The model under review builds one solid part; all positions refer to its coordinate system, in mm. A direction names the side the tool comes from. Round coordinates to 2 decimals unless told otherwise and drop trailing zeros. Order: outer loops, then holes, each group sorted by start corner. A loop starts at its lowest first (then second) coordinate and runs counter-clockwise, first axis right, second up. Notation, with made-up numbers: M -24,2.5 L 9,2.5 A23 cw 9,39.5 Z; hole C -8,76.5 d2. An arc over 180 degrees is marked long. Answer as a JSON object with one key per item and string values. Group by question number.
1. Add section A-A on z = 0.5. State the section outline as (x, y) points.
2. Clearance check with flat-ended pins moving along their axes: P1, Ø1.5, axis at x = 0, y = 12.73, coming from the +Z side; P2, Ø6.5, axis at x = -0.5, y = 20.5, coming from the +Z side. State where each tip first meets the part, or that it passes through.
3. Machinability: for faces 1 (the face through (0.02, 10.39, -3.64)), 2 (the face through (3.53, 16.46, 0.04)), 3 (the face through (-0.1, -16, 2.7)), which of the approach directions +Z, -Z, +X, -X, +Y, -Y give a long, thin tool a straight path to every point of the face, cutting with its end or side? Answer none if there is none.
4. Mouldability with a two-part tool opening along Z and no side actions: class faces 4 (the face through (0.042, -4.865, -3.635)), 5 (the face through (3.54, -16.47, 0.04)), 6 (the face through (-0.16, -11.49, -3.25)), 7 (the face through (-4, -4, -3)) as released by +Z, released by -Z, zero draft, split by the parting line, or undercut.
5. To check wall thickness, follow probe 1 along Z at (x, y) = (-12.5, 2); probe 2 along X at (y, z) = (-20, 2.9); probe 3 along Y at (x, z) = (13, -3.5). State the ranges of each line that lie inside material, in increasing order. Write a range as [from, to].
6. Add section C-C on x = 0. Give the number of separate pieces and of enclosed holes in the cut face, and give its area (3 significant figures).
7. Add section B-B on x = -7. State the section outline as (y, z) points, and give its area (3 significant figures).
```python
from build123d import *

# Parameters (mm, degrees)
SKETCH_1_R               = 1.25
SKETCH_1_R_2             = 1.5
EXTRUDE_1_DEPTH          = 4
SKETCH_2_R               = 4
CUT_EXTRUDE_1_DEPTH      = 31.055705855
CHAMFER_1_SIZE           = 0.5
SKETCH_3_R               = 5
CUT_EXTRUDE_2_DEPTH      = 2.5
CUT_EXTRUDE_4_DEPTH      = 30.246289584
CUT_EXTRUDE_4_DEPTH_BACK = 30.246289584
SKETCH_7_W               = 6
SKETCH_7_H               = 32


with BuildPart() as part:
    # 草图1 → 凸台-拉伸1 (new, symmetric)
    with BuildSketch(Plane.XY):
        with BuildLine():
            Line((-4, 20), (-4, 6.5))
            Line((-4, 6.5), (-13.804568476, 3.330290152))
            ThreePointArc((-13.804568476, 3.330290152), (-16.227922061, 0), (-13.804568476, -3.330290152))
            Line((-13.804568476, -3.330290152), (-4, -6.5))
            Line((-4, -6.5), (-4, -20))
            ThreePointArc((-4, -20), (0, -24), (4, -20))
            Line((4, -20), (4, -6.5))
            Line((4, -6.5), (13.804568476, -3.330290152))
            ThreePointArc((13.804568476, -3.330290152), (16.227922061, 0), (13.804568476, 3.330290152))
            Line((13.804568476, 3.330290152), (4, 6.5))
            Line((4, 6.5), (4, 20))
            ThreePointArc((4, 20), (0, 24), (-4, 20))
        make_face()
        with Locations((0, 12.727922061)):
            Circle(SKETCH_1_R, mode=Mode.SUBTRACT)
        with Locations((0, -12.727922061)):
            Circle(SKETCH_1_R, mode=Mode.SUBTRACT)
        with Locations((-12.727922061, 0)):
            Circle(SKETCH_1_R, mode=Mode.SUBTRACT)
        with Locations((12.727922061, 0)):
            Circle(SKETCH_1_R, mode=Mode.SUBTRACT)
        with Locations((0, 20)):
            Circle(SKETCH_1_R_2, mode=Mode.SUBTRACT)
        with Locations((0, -20)):
            Circle(SKETCH_1_R_2, mode=Mode.SUBTRACT)
    extrude(amount=EXTRUDE_1_DEPTH, both=True)

    # 草图2 → 切除-拉伸1 (cut, through all)
    with BuildSketch(Plane.XY.offset(4)):
        Circle(SKETCH_2_R)
        with BuildLine():
            Line((-0.726184377, 9.6875), (-1.452368755, 6.875))
            ThreePointArc((-1.452368755, 6.875), (0, 5), (1.452368755, 6.875))
            Line((1.452368755, 6.875), (0.726184377, 9.6875))
            ThreePointArc((0.726184377, 9.6875), (0, 10.25), (-0.726184377, 9.6875))
        make_face()
        with BuildLine():
            Line((-0.726184377, -9.6875), (-1.452368755, -6.875))
            ThreePointArc((-1.452368755, -6.875), (0, -5), (1.452368755, -6.875))
            Line((1.452368755, -6.875), (0.726184377, -9.6875))
            ThreePointArc((0.726184377, -9.6875), (0, -10.25), (-0.726184377, -9.6875))
        make_face()
    extrude(amount=-CUT_EXTRUDE_1_DEPTH, mode=Mode.SUBTRACT)

    # 倒角1
    chamfer_1_edges = [part.edges().sort_by_distance(p)[0] for p in [
        (-1.25, 12.727922061, -4),
        (-1.25, 12.727922061, 4),
        (-1.25, -12.727922061, -4),
        (-1.25, -12.727922061, 4),
        (-1.5, 20, -4),
        (-1.5, 20, 4),
        (11.477922061, 0, -4),
        (11.477922061, 0, 4),
        (-13.977922061, 0, -4),
        (-13.977922061, 0, 4),
        (-1.5, -20, -4),
        (-1.5, -20, 4),
        (0, 10.25, -4),
        (1.089276566, 8.28125, -4),
        (0, 5, -4),
        (-1.089276566, 8.28125, -4),
        (0, 10.25, 4),
        (-1.089276566, 8.28125, 4),
        (0, 5, 4),
        (1.089276566, 8.28125, 4),
        (0, -5, -4),
        (1.089276566, -8.28125, -4),
        (0, -10.25, -4),
        (-1.089276566, -8.28125, -4),
        (0, -5, 4),
        (-1.089276566, -8.28125, 4),
        (0, -10.25, 4),
        (1.089276566, -8.28125, 4),
        (-4, 0, -4),
        (-4, 0, 4),
    ]]
    chamfer(chamfer_1_edges, length=CHAMFER_1_SIZE - 0.0001)  # a hair under: the kernel refuses the full size

    # 草图3 → 切除-拉伸2 (cut, symmetric)
    with BuildSketch(Plane.XY):
        with Locations((0, 20)):
            Circle(SKETCH_3_R)
        with Locations((0, -20)):
            Circle(SKETCH_3_R)
    extrude(amount=CUT_EXTRUDE_2_DEPTH, both=True, mode=Mode.SUBTRACT)

    # 草图7 → 切除-拉伸4 (cut, two sides: drawn at the far end of the back side and taken through both)
    with BuildSketch(Plane(origin=(0, 0, 0), x_dir=(0, 0, -1), z_dir=(1, 0, 0)).offset(-CUT_EXTRUDE_4_DEPTH_BACK)):
        Rectangle(SKETCH_7_W, SKETCH_7_H)
    extrude(amount=CUT_EXTRUDE_4_DEPTH + CUT_EXTRUDE_4_DEPTH_BACK, mode=Mode.SUBTRACT)


solid = part.part
```
Recorded:
{
 "1": {"outline": "M -4,-17 A5 cw -3,-16 L -4,-16 Z; M -4,16 L -3,16 A5 cw -4,17 Z; M 3,-16 A5 cw 4,-17 L 4,-16 Z; M 3,16 L 4,16 L 4,17 A5 cw Z"},
 "2": {"P1": "passes through", "P2": "stops at z = 4"},
 "3": {"face 1": "-Z", "face 2": "+Y", "face 3": "+X, -X"},
 "4": {"face 4": "released by -Z", "face 5": "undercut", "face 6": "zero draft", "face 7": "undercut"},
 "5": {"probe 1": "z = [-4, -3], [3, 4]", "probe 2": "x = [-4, -1.5], [1.5, 4]", "probe 3": "y = [-3.59, -1.22], [1.22, 3.59]"},
 "6": {"separate pieces": "16", "enclosed holes": "0", "area": "43.5 mm²"},
 "7": {"outline": "M -5.53,-4 L 5.53,-4 L 5.53,-3 L -5.53,-3 Z; M -5.53,3 L 5.53,3 L 5.53,4 L -5.53,4 Z", "area": "22.1 mm²"}
}
